Source: CAD feature listing. Evaluate the final solid. Frame: model axes, mm. Face numbers are marked on the shaded views. Round coordinates to 2 decimals unless told otherwise and drop trailing zeros. Loops run counter-clockwise (first coordinate to the right, second up) from the corner with the lowest first, then second, coordinate; pieces in that order, holes last.
(1) Section C-C, the plane y = 1. Return the cut outline in (x, z).
(2) Section B-B, the plane y = 11. Return the cut outline in (x, z), plus the area to 3 significant figures.
(3) First-contact query: pin 1 Ø3 at (y, z) = (-17.5, 15) entering from -X; pin 2 Ø6 at (x, z) = (40, 15) entering from -Y; pin 3 Ø5 at (y, z) = (23.5, 6) entering from -X; pin 4 Ø2 at (x, y) = (25, -2.5) entering from +Z. Flat tips, straight axial feed; report the tip coordinate or a pass-through.
(4) Mould query, pull axis Y, two halves, no side actions, for the marked faces 1, 2 and 3. Classes: pulls with the +Y half, pulls with the -Y half, needs draft (parallel to the pull), parting line crosses it, or undercut.
(5) Material intervals for probe 1 along Z at (x, y) = (52.5, 22.5); probe 2 along Y at (x, z) = (0, 0.85); probe 3 along X at (y, z) = (-14.5, 18.25), sorted ascending.
(6) Section A-A, the plane x = -40. Return the cut outline in (y, z), plus the area to 3 significant figures.
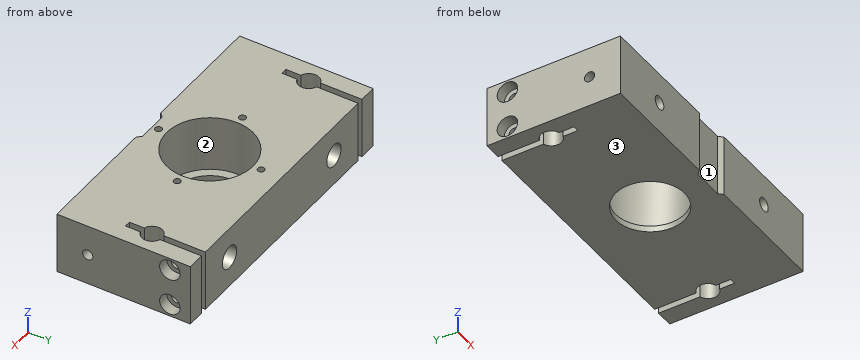
```python
from build123d import *

# Parameters (mm, degrees)
SKETCH1_W                                           = 140
SKETCH1_H                                           = 65
BOSS_EXTRUDE1_DEPTH                                 = 30
SKETCH2_R                                           = 21
CUT_EXTRUDE2_DEPTH                                  = 27
SKETCH4_R                                           = 16.75
CUT_EXTRUDE3_DEPTH                                  = 82.76337811
SKETCH5_R                                           = 5
CUT_EXTRUDE4_DEPTH                                  = 83.802475808
SKETCH6_W                                           = 3
SKETCH6_H                                           = 37
CUT_EXTRUDE5_DEPTH                                  = 83.802475808
CBORE_FOR_M5_HEX_SOCKET_HEAD_CAP_SCREW1_D           = 5.5
CBORE_FOR_M5_HEX_SOCKET_HEAD_CAP_SCREW1_DEPTH       = 8.5
CBORE_FOR_M5_HEX_SOCKET_HEAD_CAP_SCREW1_CBORE_D     = 10
CBORE_FOR_M5_HEX_SOCKET_HEAD_CAP_SCREW1_CBORE_DEPTH = 5.4
TAP_DRILL_FOR_M5_TAP1_AT_2_COUNT                    = 2
TAP_DRILL_FOR_M5_TAP1_AT_2_PITCH                    = 18
CBORE_FOR_M6_HEX_SOCKET_HEAD_CAP_SCREW3_D           = 6.6
CBORE_FOR_M6_HEX_SOCKET_HEAD_CAP_SCREW3_CBORE_D     = 11
CBORE_FOR_M6_HEX_SOCKET_HEAD_CAP_SCREW3_CBORE_DEPTH = 61.4
CIRPATTERN1_COUNT                                   = 4
SKETCH29_W                                          = 35
SKETCH29_H                                          = 2
CUT_EXTRUDE6_DEPTH                                  = 83.802475808
CHAMFER2_SIZE                                       = 10


with BuildPart() as part:
    # Sketch1 → Boss-Extrude1 (new body)
    with BuildSketch(Plane.XY):
        Rectangle(SKETCH1_W, SKETCH1_H)
    extrude(amount=BOSS_EXTRUDE1_DEPTH)

    # Sketch2 → Cut-Extrude2 (cut)
    with BuildSketch(Plane(origin=(0, 0, 30), x_dir=(-1, 0, 0), z_dir=(0, 0, -1))):
        with Locations((0, -2.5)):
            Circle(SKETCH2_R)
    extrude(amount=CUT_EXTRUDE2_DEPTH, mode=Mode.SUBTRACT)

    # Sketch4 → Cut-Extrude3 (cut, through all)
    with BuildSketch(Plane.XY.offset(3)):
        with Locations((0, -2.5)):
            Circle(SKETCH4_R)
    extrude(amount=-CUT_EXTRUDE3_DEPTH, mode=Mode.SUBTRACT)

    # Sketch5 → Cut-Extrude4 (cut, through all)
    with BuildSketch(Plane(origin=(0, 0, 0), x_dir=(-1, 0, 0), z_dir=(0, 0, -1))):
        with Locations((-60, 7.5)):
            Circle(SKETCH5_R)
        with Locations((60, 7.5)):
            Circle(SKETCH5_R)
    extrude(amount=-CUT_EXTRUDE4_DEPTH, mode=Mode.SUBTRACT)

    # Sketch6 → Cut-Extrude5 (cut, through all)
    with BuildSketch(Plane(origin=(0, 0, 0), x_dir=(-1, 0, 0), z_dir=(0, 0, -1))):
        with Locations((-60, 14)):
            Rectangle(SKETCH6_W, SKETCH6_H)
        with Locations((60, 14)):
            Rectangle(SKETCH6_W, SKETCH6_H)
    extrude(amount=-CUT_EXTRUDE5_DEPTH, mode=Mode.SUBTRACT)

    # CBORE for M5 Hex Socket Head Cap Screw1
    with Locations(Plane(origin=(70, 0, 0), x_dir=(0, 0, -1), z_dir=(1, 0, 0))):
        with Locations((-6, 22.5), (-24, 22.5)):
            cbore_for_m5_hex_socket_head_cap_screw1 = CounterBoreHole(CBORE_FOR_M5_HEX_SOCKET_HEAD_CAP_SCREW1_D / 2, CBORE_FOR_M5_HEX_SOCKET_HEAD_CAP_SCREW1_CBORE_D / 2, CBORE_FOR_M5_HEX_SOCKET_HEAD_CAP_SCREW1_CBORE_DEPTH, depth=CBORE_FOR_M5_HEX_SOCKET_HEAD_CAP_SCREW1_DEPTH)

    # Sketch12 → Tap Drill for M5 Tap1 (revolve, cut)
    with BuildSketch(Plane(origin=(58.5, 22.5, 6), x_dir=(0, 0, -1), z_dir=(0, 1, 0))):
        Polygon((0, 0), (0, 13.2618073), (2.1, 12), (2.1, 0), align=None)
    tap_drill_for_m5_tap1 = revolve(axis=Axis((64.85, 22.5, 6), (-1, 0, 0)), mode=Mode.SUBTRACT)

    # Tap Drill for M5 Tap1 at 2: Tap Drill for M5 Tap1 ×2
    with Locations(*[(0, 0, i * TAP_DRILL_FOR_M5_TAP1_AT_2_PITCH) for i in range(1, TAP_DRILL_FOR_M5_TAP1_AT_2_COUNT)]):
        add(tap_drill_for_m5_tap1, mode=Mode.SUBTRACT)

    # Sketch15 → Tap Drill for M6 Tap1 (revolve, cut)
    with BuildSketch(Plane(origin=(70, -17.5, 15), x_dir=(0, 0, -1), z_dir=(0, 1, 0))):
        Polygon((0, 0), (0, 16.502151548), (2.5, 15), (2.5, 0), align=None)
    tap_drill_for_m6_tap1 = revolve(axis=Axis((76.35, -17.5, 15), (-1, 0, 0)), mode=Mode.SUBTRACT)

    # Mirror1: CBORE for M5 Hex Socket Head Cap Screw1, Tap Drill for M5 Tap1, Tap Drill for M6 Tap1 across plane
    add(cbore_for_m5_hex_socket_head_cap_screw1.mirror(Plane(origin=(0, 0, 0), x_dir=(0, 0, 1), z_dir=(1, 0, 0))), mode=Mode.SUBTRACT)
    add(tap_drill_for_m5_tap1.mirror(Plane(origin=(0, 0, 0), x_dir=(0, 0, 1), z_dir=(1, 0, 0))), mode=Mode.SUBTRACT)
    add(tap_drill_for_m6_tap1.mirror(Plane(origin=(0, 0, 0), x_dir=(0, 0, 1), z_dir=(1, 0, 0))), mode=Mode.SUBTRACT)

    # Mirror1 copy 1 sketch → Mirror1 copy 1 (revolve, cut)
    with BuildSketch(Plane(origin=(-58.5, 22.5, 24), x_dir=(0, 0, -1), z_dir=(0, 1, 0))):
        Polygon((0, 0), (0, -13.2618073), (2.1, -12), (2.1, 0), align=None)
    revolve(axis=Axis((-64.85, 22.5, 24), (-1, 0, 0)), mode=Mode.SUBTRACT)

    # CBORE for M6 Hex Socket Head Cap Screw3 (through all)
    with Locations(Plane(origin=(0, 32.5, 0), x_dir=(1, 0, 0), z_dir=(0, 1, 0))):
        with Locations((40, -15), (-40, -15)):
            CounterBoreHole(CBORE_FOR_M6_HEX_SOCKET_HEAD_CAP_SCREW3_D / 2, CBORE_FOR_M6_HEX_SOCKET_HEAD_CAP_SCREW3_CBORE_D / 2, CBORE_FOR_M6_HEX_SOCKET_HEAD_CAP_SCREW3_CBORE_DEPTH)

    # Sketch28 → Tap Drill for M4 Tap1 (revolve, cut)
    with BuildSketch(Plane(origin=(0, 22.5, 30), x_dir=(0, -1, 0), z_dir=(1, 0, 0))):
        Polygon((0, 0), (0, 8.991420021), (1.65, 8), (1.65, 0), align=None)
    tap_drill_for_m4_tap1 = revolve(axis=Axis((0, 22.5, 36.35), (0, 0, -1)), mode=Mode.SUBTRACT)

    # CirPattern1: Tap Drill for M4 Tap1 ×4 about axis
    cirpattern1_axis = Axis((0, -2.5, 0), (0, 0, 1))
    for i in range(1, CIRPATTERN1_COUNT):
        add(tap_drill_for_m4_tap1.rotate(cirpattern1_axis, i * 360 / CIRPATTERN1_COUNT), mode=Mode.SUBTRACT)

    # Sketch29 → Cut-Extrude6 (cut, through all)
    with BuildSketch(Plane.XY.offset(30)):
        with Locations((0, -31.5)):
            Rectangle(SKETCH29_W, SKETCH29_H)
    extrude(amount=-CUT_EXTRUDE6_DEPTH, mode=Mode.SUBTRACT)

    # Chamfer2
    # the kernel refuses this chamfer: 10 mm, written as the material it adds along each edge
    with BuildSketch(Plane(origin=(-17.5, -30.5, 30), x_dir=(-0.02749587661058977, -0.9996219169112965, 0), z_dir=(0, 0, -1))) as chamfer2_piece_1_section:
        Polygon((CHAMFER2_SIZE * 0.999621916911, -CHAMFER2_SIZE * 0.0274958766106), (-CHAMFER2_SIZE * 0.0274958766106, -CHAMFER2_SIZE * 0.999621916911), (0, 0), align=None)
    chamfer2_piece_1 = extrude(amount=30, mode=Mode.PRIVATE)
    chamfer2_piece_1 = split(chamfer2_piece_1, bisect_by=Plane(origin=(-12.880949734, -32.5, 15), z_dir=(0, 1, 0)), keep=Keep.TOP, mode=Mode.PRIVATE)
    add(chamfer2_piece_1)
    with BuildSketch(Plane(origin=(17.5, -30.5, 30), x_dir=(-0.9996219169112968, 0.027495876610586317, 0), z_dir=(0, 0, -1))) as chamfer2_piece_2_section:
        Polygon((CHAMFER2_SIZE * 0.999621916911, -CHAMFER2_SIZE * 0.0274958766106), (-CHAMFER2_SIZE * 0.0274958766106, -CHAMFER2_SIZE * 0.999621916911), (0, 0), align=None)
    chamfer2_piece_2 = extrude(amount=30, mode=Mode.PRIVATE)
    chamfer2_piece_2 = split(chamfer2_piece_2, bisect_by=Plane(origin=(12.880949734, -32.5, 15), z_dir=(0, 1, 0)), keep=Keep.TOP, mode=Mode.PRIVATE)
    add(chamfer2_piece_2)


solid = part.part
```
Output values:
1. outline: (-70, 0) - (-61.5, 0) - (-61.5, 30) - (-70, 30) - close; (-58.5, 0) - (-16.38, 0) - (-16.38, 3) - (-20.71, 3) - (-20.71, 30) - (-58.5, 30) - close; (16.38, 0) - (58.5, 0) - (58.5, 30) - (20.71, 30) - (20.71, 3) - (16.38, 3) - close; (61.5, 0) - (70, 0) - (70, 30) - (61.5, 30) - close; hole circle Ø11 at (-40, 15); hole circle Ø11 at (40, 15)
2. outline: (-70, 0) - (-63.57, 0) - (-63.57, 30) - (-70, 30) - close; (-56.43, 0) - (-9.92, 0) - (-9.92, 3) - (-16.09, 3) - (-16.09, 30) - (-56.43, 30) - close; (9.92, 0) - (56.43, 0) - (56.43, 30) - (16.09, 30) - (16.09, 3) - (9.92, 3) - close; (63.57, 0) - (70, 0) - (70, 30) - (63.57, 30) - close; hole circle Ø11 at (-40, 15); hole circle Ø11 at (40, 15)
2. area: 2,650 mm2
3. pin 1: stops at x = -54.4
3. pin 2: passes through
3. pin 3: stops at x = -64.6
3. pin 4: stops at z = 21.61
4. face 1: pulls with the -Y half
4. face 2: undercut
4. face 3: needs draft
5. probe 1: z = 0 to 3.9, 8.1 to 21.9, 26.1 to 30
5. probe 2: y = -30.5 to -19.25, 14.25 to 32.5
5. probe 3: x = -70 to -44.44, -35.56 to -17.23, 17.23 to 35.56, 44.44 to 70
6. outline: (-32.5, 0) - (32.5, 0) - (32.5, 9.5) - (-28.9, 9.5) - (-28.9, 11.7) - (-32.5, 11.7) - close; (-32.5, 18.3) - (-28.9, 18.3) - (-28.9, 20.5) - (32.5, 20.5) - (32.5, 30) - (-32.5, 30) - close
6. area: 1,250 mm2
